```python
from build123d import *

# Parameters (mm, degrees)
SKETCH1_W           = 38.1
SKETCH1_H           = 38.1
BOSS_EXTRUDE1_DEPTH = 5.08
SKETCH5_W           = 2.032
SKETCH5_H           = 33.02
BOSS_EXTRUDE3_DEPTH = 2.54
SKETCH6_W           = 22.86
SKETCH6_H           = 5.08
CUT_EXTRUDE1_DEPTH  = 8.62
FILLET1_R           = 1.27


with BuildPart() as part:
    # Sketch1 → Boss-Extrude1 (new body)
    with BuildSketch(Plane.XY):
        with Locations((0.962710567, -6.301378254)):
            Rectangle(SKETCH1_W, SKETCH1_H)
    extrude(amount=BOSS_EXTRUDE1_DEPTH)

    # Sketch5 → Boss-Extrude3 (add)
    with BuildSketch(Plane.XY.offset(5.08)):
        with Locations((14.686710567, -6.301378254)):
            Rectangle(SKETCH5_W, SKETCH5_H)
        with Locations((-12.761289417, -6.301378254)):
            Rectangle(SKETCH5_W, SKETCH5_H)
    extrude(amount=BOSS_EXTRUDE3_DEPTH)

    # Sketch6 → Cut-Extrude1 (cut, through all)
    with BuildSketch(Plane(origin=(0, 0, 0), x_dir=(-1, 0, 0), z_dir=(0, 0, -1))):
        with Locations((-0.962710567, 10.208621746)):
            Rectangle(SKETCH6_W, SKETCH6_H)
        with Locations((-0.962710567, -22.811378254)):
            Rectangle(SKETCH6_W, SKETCH6_H)
    extrude(amount=-CUT_EXTRUDE1_DEPTH, mode=Mode.SUBTRACT)

    # Fillet1
    fillet1_edges = [part.edges().sort_by_distance(p)[0] for p in [
        (-14.277289433, 12.748621746, 0),
        (16.202710567, -25.351378254, 0),
        (16.202710567, 12.748621746, 0),
        (20.012710567, -6.301378254, 0),
        (-10.467289433, 10.208621746, 0),
        (12.392710567, 10.208621746, 0),
        (0.962710567, 7.668621746, 0),
        (-14.277289433, -25.351378254, 0),
        (-18.087289433, -6.301378254, 0),
        (12.392710567, -22.811378254, 0),
        (-10.467289433, -22.811378254, 0),
        (0.962710567, -20.271378254, 0),
    ]]
    fillet(fillet1_edges, radius=FILLET1_R)


solid = part.part
```
Input: part model. Units: mm. Frame: model coordinates. A direction names the side the tool comes from. Round coordinates to 2 decimals unless told otherwise and drop trailing zeros. Loops run counter-clockwise (first coordinate to the right, second up) from the corner with the lowest first, then second, coordinate; pieces in that order, holes last. Notation, with made-up numbers: (-26, 76.5) -> (10, 76.5) arc R15 cw to (10, 94.5) -> close; hole circle Ø9 at (-28.5, 16). An arc over 180 degrees is marked (long way). Use one line per item in the form item = value. Start each with the question number.
Item 1: Section query D-D on x = -12.5. Return the cut outline in (y, z).
Item 2: Section query B-B on z = 2. Return the cut outline in (x, y), then the cut area to 3 significant figures.
Item 3: Mould query, pull axis X, two halves, no side actions, for faces 1 (the face through (15, -6, 7.62)), 2 (the face through (19.63, -6.03, 0.36)), 3 (the face through (0.785, 7.287, 0.362)). Classes: pulls with the +X half, pulls with the -X half, needs draft (parallel to the pull), parting line crosses it, or undercut.
Item 4: Contact query for flat-ended pins moving along their axis: pin 1 Ø1.3 at (y, z) = (1, 6) entering from -X; pin 2 Ø1.6 at (x, z) = (-13, 6.5) entering from -Y; pin 3 Ø1 at (x, z) = (-12.5, 6.5) entering from +Y. Output: stop coordinate, or through.
Item 5: Material intervals for L1, parallel to X at y = -7, z = 5.5; L2, parallel to Y at x = 4.5, z = 2.5; L3, parallel to Z at x = -6, y = 2, sorted ascending. Write a range as from..to.
Item 6: Section query C-C on y = -16.5. Return the cut outline in (x, z).
Item 7: Section query A-A on y = -22. Return the cut outline in (x, z), then the cut area to 3 significant figures.
Item 8: Set-up query: faces 4 (the face through (-13, -22.811, 6)), 5 (the face through (0.78, -19.89, 0.36)), 6 (the face through (12.775, 9.618, 0.362)). Return all of +Z, -Z, +X, -X, +Y, -Y with unobstructed straight access to the full face (end or side cutting, diameter ignored); none if empty.
Ans:
q1.outline = (-25.35, 1.27) arc R1.27 ccw to (-24.08, 0) -> (11.48, 0) arc R1.27 ccw to (12.75, 1.27) -> (12.75, 5.08) -> (10.21, 5.08) -> (10.21, 7.62) -> (-22.81, 7.62) -> (-22.81, 5.08) -> (-25.35, 5.08) -> close
q2.outline = (-18.09, -25.35) -> (-10.47, -25.35) -> (-10.47, -20.27) -> (12.39, -20.27) -> (12.39, -25.35) -> (20.01, -25.35) -> (20.01, 12.75) -> (12.39, 12.75) -> (12.39, 7.67) -> (-10.47, 7.67) -> (-10.47, 12.75) -> (-18.09, 12.75) -> close
q2.area = 1,220 mm^2
q3.face_1 = needs draft
q3.face_2 = pulls with the +X half
q3.face_3 = undercut
q4.pin_1 = -13.78
q4.pin_2 = -22.81
q4.pin_3 = 10.21
q5.L1 = -13.78..-11.75, 13.67..15.7
q5.L2 = -20.27..7.67
q5.L3 = 0..5.08
q6.outline = (-18.09, 1.27) arc R1.27 ccw to (-16.82, 0) -> (18.74, 0) arc R1.27 ccw to (20.01, 1.27) -> (20.01, 5.08) -> (15.7, 5.08) -> (15.7, 7.62) -> (13.67, 7.62) -> (13.67, 5.08) -> (-11.75, 5.08) -> (-11.75, 7.62) -> (-13.78, 7.62) -> (-13.78, 5.08) -> (-18.09, 5.08) -> close
q7.outline = (-18.09, 1.27) arc R1.27 ccw to (-16.82, 0) -> (-11.74, 0) arc R1.27 ccw to (-10.47, 1.27) -> (-10.47, 5.08) -> (-11.75, 5.08) -> (-11.75, 7.62) -> (-13.78, 7.62) -> (-13.78, 5.08) -> (-18.09, 5.08) -> close; (12.39, 1.27) arc R1.27 ccw to (13.66, 0) -> (18.74, 0) arc R1.27 ccw to (20.01, 1.27) -> (20.01, 5.08) -> (15.7, 5.08) -> (15.7, 7.62) -> (13.67, 7.62) -> (13.67, 5.08) -> (12.39, 5.08) -> close
q7.area = 86.4 mm^2
q8.face_4 = +Z, +X, -X, -Y
q8.face_5 = -Z, -Y
q8.face_6 = -Z, +Y
